from build123d import *

# Parameters (mm, degrees)
AUFSATZ_LINEAR_AUSTRAGEN1_DEPTH  = 67
SKIZZE3_W                        = 151
SKIZZE3_H                        = 2
AUFSATZ_LINEAR_AUSTRAGEN2_DEPTH  = 47.34238026
SKIZZE4_W                        = 2
SKIZZE4_H                        = 65
AUFSATZ_LINEAR_AUSTRAGEN3_DEPTH  = 47.39811
SKIZZE6_W                        = 149
SKIZZE6_H                        = 2
AUFSATZ_LINEAR_AUSTRAGEN4_DEPTH  = 47.40101983
SKIZZE7_W                        = 2
SKIZZE7_H                        = 63
AUFSATZ_LINEAR_AUSTRAGEN5_DEPTH  = 47.37320267
SKIZZE20_W                       = 147
SKIZZE20_H                       = 12.080237494
AUFSATZ_LINEAR_AUSTRAGEN6_DEPTH  = 63
SCHNITT_LINEAR_AUSTRAGEN1_DEPTH  = 137.764615455
SKIZZE23_W                       = 7.8
SKIZZE23_H                       = 5.4
SCHNITT_LINEAR_AUSTRAGEN12_DEPTH = 47
SKIZZE26_R                       = 2.05
SCHNITT_LINEAR_AUSTRAGEN13_DEPTH = 38
SKIZZE28_R                       = 2.05
SCHNITT_LINEAR_AUSTRAGEN14_DEPTH = 38
SCHNITT_LINEAR_START             = -38
SKIZZE29_R                       = 2.05
SCHNITT_LINEAR_AUSTRAGEN15_DEPTH = 38
SKIZZE31_R                       = 2.05
SCHNITT_LINEAR_AUSTRAGEN16_DEPTH = 38
SKIZZE32_R                       = 3
AUFSATZ_LINEAR_AUSTRAGEN15_DEPTH = 23.29
SKIZZE33_R                       = 3
AUFSATZ_LINEAR_AUSTRAGEN16_DEPTH = 23.29
SKIZZE34_R                       = 1.65
SCHNITT_LINEAR_AUSTRAGEN17_DEPTH = 25
SKIZZE35_R                       = 1.65
SCHNITT_LINEAR_AUSTRAGEN18_DEPTH = 25
SKIZZE37_W                       = 67
SKIZZE37_H                       = 9
SCHNITT_LINEAR_AUSTRAGEN20_DEPTH = 6.5
SKIZZE38_W                       = 67
SKIZZE38_H                       = 9
SCHNITT_LINEAR_AUSTRAGEN21_DEPTH = 6.5
FASE2_SIZE                       = 1
FASE13_SIZE                      = 1
SKIZZE40_R                       = 2.85
AUFSATZ_LINEAR_AUSTRAGEN17_DEPTH = 1.5
SKIZZE41_R                       = 1.65
SCHNITT_LINEAR_AUSTRAGEN23_DEPTH = 5
SKIZZE42_R                       = 2.85
AUFSATZ_LINEAR_AUSTRAGEN18_DEPTH = 1.5
SCHNITT_LINEAR_AUSTRAGEN24_DEPTH = 2
SKIZZE46_W                       = 5
SKIZZE46_H                       = 2.5
AUFSATZ_LINEAR_AUSTRAGEN21_DEPTH = 5
SKIZZE47_W                       = 5
SKIZZE47_H                       = 2.5
AUFSATZ_LINEAR_AUSTRAGEN22_DEPTH = 5
SKIZZE48_W                       = 38
SKIZZE48_H                       = 20.6
SCHNITT_LINEAR_AUSTRAGEN25_DEPTH = 2
SKIZZE49_W                       = 38
SKIZZE49_H                       = 2
AUFSATZ_LINEAR_AUSTRAGEN23_DEPTH = 10
SKIZZE51_R                       = 3
AUFSATZ_LINEAR_AUSTRAGEN24_DEPTH = 2.5
SKIZZE52_R                       = 1.6
SCHNITT_LINEAR_AUSTRAGEN26_DEPTH = 15


with BuildPart() as part:
    # Skizze1 → Aufsatz-Linear austragen1 (new body)
    with BuildSketch(Plane.XY):
        with BuildLine():
            Line((13.401569275, 0), (13.401569275, -2))
            Line((13.401569275, -2), (53.401569275, -2))
            Line((53.401569275, -2), (53.401569275, 0))
            ThreePointArc((53.401569275, 0), (63.401569275, 10), (73.401569275, 0))
            Line((73.401569275, 0), (73.401569275, -2))
            Line((73.401569275, -2), (109.401569275, -2))
            Line((109.401569275, -2), (109.401569275, 0))
            Line((109.401569275, 0), (75.401569275, 0))
            ThreePointArc((75.401569275, 0), (63.401569275, 12), (51.401569275, 0))
            Line((51.401569275, 0), (15.488199501, 0))
            ThreePointArc((15.488199501, 0), (3.901569275, 8.877501001), (-7.685060952, 0))
            Line((-7.685060952, 0), (-41.598430725, 0))
            Line((-41.598430725, 0), (-41.598430725, -2))
            Line((-41.598430725, -2), (-5.598430725, -2))
            Line((-5.598430725, -2), (-5.598430725, 0))
            ThreePointArc((-5.598430725, 0), (3.901569275, 6.877501001), (13.401569275, 0))
        make_face()
    extrude(amount=AUFSATZ_LINEAR_AUSTRAGEN1_DEPTH)

    # Skizze3 → Aufsatz-Linear austragen2 (add)
    with BuildSketch(Plane(origin=(0, 0, 0), x_dir=(1, 0, 0), z_dir=(0, 1, 0))):
        with Locations((33.901569275, -1)):
            Rectangle(SKIZZE3_W, SKIZZE3_H)
    extrude(amount=AUFSATZ_LINEAR_AUSTRAGEN2_DEPTH)

    # Skizze4 → Aufsatz-Linear austragen3 (add)
    with BuildSketch(Plane(origin=(0, 0, 0), x_dir=(1, 0, 0), z_dir=(0, 1, 0))):
        with Locations((-40.598430725, -34.5)):
            Rectangle(SKIZZE4_W, SKIZZE4_H)
    extrude(amount=AUFSATZ_LINEAR_AUSTRAGEN3_DEPTH)

    # Skizze6 → Aufsatz-Linear austragen4 (add)
    with BuildSketch(Plane(origin=(0, 0, 0), x_dir=(1, 0, 0), z_dir=(0, 1, 0))):
        with Locations((34.901569275, -66)):
            Rectangle(SKIZZE6_W, SKIZZE6_H)
    extrude(amount=AUFSATZ_LINEAR_AUSTRAGEN4_DEPTH)

    # Skizze7 → Aufsatz-Linear austragen5 (add)
    with BuildSketch(Plane(origin=(0, 0, 0), x_dir=(1, 0, 0), z_dir=(0, 1, 0))):
        with Locations((108.401569275, -33.5)):
            Rectangle(SKIZZE7_W, SKIZZE7_H)
    extrude(amount=AUFSATZ_LINEAR_AUSTRAGEN5_DEPTH)

    # Skizze20 → Aufsatz-Linear austragen6 (add)
    with BuildSketch(Plane.XY.offset(2)):
        with Locations((33.901569275, 6.040118747)):
            Rectangle(SKIZZE20_W, SKIZZE20_H)
    extrude(amount=AUFSATZ_LINEAR_AUSTRAGEN6_DEPTH)

    # Skizze8 → Schnitt-Linear austragen1 (cut, through all)
    with BuildSketch(Plane.XY.offset(67)):
        with BuildLine():
            Line((53.401569275, 0), (73.401569275, 0))
            ThreePointArc((73.401569275, 0), (63.401569275, 10), (53.401569275, 0))
        make_face()
        with BuildLine():
            Line((-5.598430725, 0), (13.401569275, 0))
            ThreePointArc((13.401569275, 0), (3.901569275, 9.5), (-5.598430725, 0))
        make_face()
    extrude(amount=-SCHNITT_LINEAR_AUSTRAGEN1_DEPTH, mode=Mode.SUBTRACT)

    # Skizze23 → Schnitt-Linear austragen12 (cut)
    with BuildSketch(Plane(origin=(109.401569275, 0, 0), x_dir=(0, 0, -1), z_dir=(1, 0, 0))):
        with Locations((-60.6, 17.280237494)):
            Rectangle(SKIZZE23_W, SKIZZE23_H)
        with Locations((-50.4, 17.280237494)):
            Rectangle(SKIZZE23_W, SKIZZE23_H)
    extrude(amount=-SCHNITT_LINEAR_AUSTRAGEN12_DEPTH, mode=Mode.SUBTRACT)

    # Skizze26 → Schnitt-Linear austragen13 (cut)
    with BuildSketch(Plane(origin=(109.401569275, 0, 0), x_dir=(0, 0, -1), z_dir=(1, 0, 0))):
        with Locations((-57, 3)):
            Circle(SKIZZE26_R)
    extrude(amount=-SCHNITT_LINEAR_AUSTRAGEN13_DEPTH, mode=Mode.SUBTRACT)

    # Skizze28 → Schnitt-Linear austragen14 (cut)
    with BuildSketch(Plane(origin=(109.401569275, 0, 0), x_dir=(0, 0, -1), z_dir=(1, 0, 0))):
        with Locations((-10, 3)):
            Circle(SKIZZE28_R)
    extrude(amount=-SCHNITT_LINEAR_AUSTRAGEN14_DEPTH, mode=Mode.SUBTRACT)

    # Skizze29 → Schnitt-Linear austragen15 (cut)
    with BuildSketch(Plane.ZY.offset(41.598430725).offset(SCHNITT_LINEAR_START)):
        with Locations(Location((57, 3, 0), (0, 0, 180))):
            Circle(SKIZZE29_R)
    extrude(amount=SCHNITT_LINEAR_AUSTRAGEN15_DEPTH, mode=Mode.SUBTRACT)

    # Skizze31 → Schnitt-Linear austragen16 (cut)
    with BuildSketch(Plane.ZY.offset(41.598430725).offset(SCHNITT_LINEAR_START)):
        with Locations(Location((10, 3, 0), (0, 0, 180))):
            Circle(SKIZZE31_R)
    extrude(amount=SCHNITT_LINEAR_AUSTRAGEN16_DEPTH, mode=Mode.SUBTRACT)

    # Skizze32 → Aufsatz-Linear austragen15 (add)
    with BuildSketch(Plane(origin=(0, 12.080237494, 0), x_dir=(1, 0, 0), z_dir=(0, 1, 0))):
        with Locations((-36.098430725, -61.5)):
            Circle(SKIZZE32_R)
    extrude(amount=AUFSATZ_LINEAR_AUSTRAGEN15_DEPTH)

    # Skizze33 → Aufsatz-Linear austragen16 (add)
    with BuildSketch(Plane(origin=(0, 12.080237494, 0), x_dir=(1, 0, 0), z_dir=(0, 1, 0))):
        with Locations((103.901569275, -5.5)):
            Circle(SKIZZE33_R)
    extrude(amount=AUFSATZ_LINEAR_AUSTRAGEN16_DEPTH)

    # Skizze34 → Schnitt-Linear austragen17 (cut)
    with BuildSketch(Plane(origin=(0, 35.370237494, 0), x_dir=(1, 0, 0), z_dir=(0, 1, 0))):
        with Locations(Location((-36.098430725, -61.5, 0), (0, 0, 180))):
            Circle(SKIZZE34_R)
    extrude(amount=-SCHNITT_LINEAR_AUSTRAGEN17_DEPTH, mode=Mode.SUBTRACT)

    # Skizze35 → Schnitt-Linear austragen18 (cut)
    with BuildSketch(Plane(origin=(0, 35.370237494, 0), x_dir=(1, 0, 0), z_dir=(0, 1, 0))):
        with Locations(Location((103.901569275, -5.5, 0), (0, 0, 180))):
            Circle(SKIZZE35_R)
    extrude(amount=-SCHNITT_LINEAR_AUSTRAGEN18_DEPTH, mode=Mode.SUBTRACT)

    # Skizze37 → Schnitt-Linear austragen20 (cut)
    with BuildSketch(Plane(origin=(109.401569275, 0, 0), x_dir=(0, 0, -1), z_dir=(1, 0, 0))):
        with Locations((-33.5, 2.5)):
            Rectangle(SKIZZE37_W, SKIZZE37_H)
    extrude(amount=-SCHNITT_LINEAR_AUSTRAGEN20_DEPTH, mode=Mode.SUBTRACT)

    # Skizze38 → Schnitt-Linear austragen21 (cut)
    with BuildSketch(Plane.ZY.offset(41.598430725)):
        with Locations((33.5, 2.5)):
            Rectangle(SKIZZE38_W, SKIZZE38_H)
    extrude(amount=-SCHNITT_LINEAR_AUSTRAGEN21_DEPTH, mode=Mode.SUBTRACT)

    # Fase2
    fase2_edges = [part.edges().sort_by_distance(p)[0] for p in [
        (-41.598430725, 27.17119013, 0),
        (109.401569275, 27.17119013, 0),
        (109.401569275, 27.200509915, 67),
        (109.401569275, 7, 33.5),
        (102.901569275, 2.5, 67),
        (106.151569275, 7, 67),
        (102.901569275, 2.5, 0),
        (106.151569275, 7, 0),
        (102.901569275, -2, 33.5),
        (-41.598430725, 7, 33.5),
        (-35.098430725, 2.5, 0),
        (-38.348430725, 7, 0),
        (-35.098430725, 2.5, 67),
        (-38.348430725, 7, 67),
        (-35.098430725, -2, 33.5),
        (-41.598430725, 27.199055, 67),
    ]]
    chamfer(fase2_edges, length=FASE2_SIZE)

    # Fase13
    fase13_edges = [part.edges().sort_by_distance(p)[0] for p in [
        (33.401569275, -2, 67),
        (87.651569275, -2, 0),
        (33.401569275, -2, 0),
        (87.651569275, -2, 67),
        (-19.848430725, -2, 0),
        (-19.848430725, -2, 67),
    ]]
    chamfer(fase13_edges, length=FASE13_SIZE)

    # Skizze40 → Aufsatz-Linear austragen17 (add)
    with BuildSketch(Plane(origin=(0, 12.080237494, 0), x_dir=(1, 0, 0), z_dir=(0, 1, 0))):
        with Locations((103.091569275, -37.57)):
            Circle(SKIZZE40_R)
    extrude(amount=AUFSATZ_LINEAR_AUSTRAGEN17_DEPTH)

    # Skizze41 → Schnitt-Linear austragen23 (cut)
    with BuildSketch(Plane(origin=(0, 13.580237494, 0), x_dir=(1, 0, 0), z_dir=(0, 1, 0))):
        with Locations(Location((103.091569275, -37.59, 0), (0, 0, 180))):
            Circle(SKIZZE41_R)
    extrude(amount=-SCHNITT_LINEAR_AUSTRAGEN23_DEPTH, mode=Mode.SUBTRACT)

    # Skizze42 → Aufsatz-Linear austragen18 (add)
    with BuildSketch(Plane(origin=(0, 12.080237494, 0), x_dir=(1, 0, 0), z_dir=(0, 1, 0))):
        with Locations((103.091569275, -60.69)):
            Circle(SKIZZE42_R)
        with Locations((68.201569275, -60.69)):
            Circle(SKIZZE42_R)
    extrude(amount=AUFSATZ_LINEAR_AUSTRAGEN18_DEPTH)

    # Skizze43 → Schnitt-Linear austragen24 (cut)
    with BuildSketch(Plane(origin=(109.401569275, 0, 0), x_dir=(0, 0, -1), z_dir=(1, 0, 0))):
        with BuildLine():
            Line((-12.5, 19.780237494), (-10.5, 19.780237494))
            ThreePointArc((-10.5, 19.780237494), (-8, 17.280237494), (-10.5, 14.780237494))
            Line((-10.5, 14.780237494), (-12.5, 14.780237494))
            ThreePointArc((-12.5, 14.780237494), (-15, 17.280237494), (-12.5, 19.780237494))
        make_face()
    extrude(amount=-SCHNITT_LINEAR_AUSTRAGEN24_DEPTH, mode=Mode.SUBTRACT)

    # Skizze46 → Aufsatz-Linear austragen21 (add)
    with BuildSketch(Plane(origin=(-39.598430725, 0, 0), x_dir=(0, 0, -1), z_dir=(1, 0, 0))):
        with Locations((-4.5, 34.120237494)):
            Rectangle(SKIZZE46_W, SKIZZE46_H)
    extrude(amount=AUFSATZ_LINEAR_AUSTRAGEN21_DEPTH)

    # Skizze47 → Aufsatz-Linear austragen22 (add)
    with BuildSketch(Plane.ZY.offset(-107.401569275)):
        with Locations((62.5, 34.120237494)):
            Rectangle(SKIZZE47_W, SKIZZE47_H)
    extrude(amount=AUFSATZ_LINEAR_AUSTRAGEN22_DEPTH)

    # Skizze48 → Schnitt-Linear austragen25 (cut)
    with BuildSketch(Plane.ZY.offset(41.598430725)):
        with Locations((33.5, 24.82)):
            Rectangle(SKIZZE48_W, SKIZZE48_H)
    extrude(amount=-SCHNITT_LINEAR_AUSTRAGEN25_DEPTH, mode=Mode.SUBTRACT)

    # Skizze49 → Aufsatz-Linear austragen23 (add)
    with BuildSketch(Plane.ZY.offset(41.598430725)):
        with Locations((33.5, 13.52)):
            Rectangle(SKIZZE49_W, SKIZZE49_H)
    extrude(amount=AUFSATZ_LINEAR_AUSTRAGEN23_DEPTH)

    # Skizze51 → Aufsatz-Linear austragen24 (add)
    with BuildSketch(Plane(origin=(0, 12.080237494, 0), x_dir=(1, 0, 0), z_dir=(0, 1, 0))):
        with Locations((-9.198430725, -29)):
            Circle(SKIZZE51_R)
    extrude(amount=AUFSATZ_LINEAR_AUSTRAGEN24_DEPTH)

    # Skizze52 → Schnitt-Linear austragen26 (cut)
    with BuildSketch(Plane(origin=(0, 14.580237494, 0), x_dir=(1, 0, 0), z_dir=(0, 1, 0))):
        with Locations(Location((-9.198430725, -29, 0), (0, 0, 180))):
            Circle(SKIZZE52_R)
    extrude(amount=-SCHNITT_LINEAR_AUSTRAGEN26_DEPTH, mode=Mode.SUBTRACT)


solid = part.part
Work out the finished part from the listing and answer in its coordinate system (mm). A direction names the side the tool comes from. Give positions to 0.01 mm unless a question says otherwise; leave off trailing zeros. Order: outer loops, then holes, each group sorted by start corner. A loop starts at its lowest first (then second) coordinate and runs counter-clockwise, first axis right, second up. Notation, with made-up numbers: (33.25, 76) -> (45.25, 76) arc R11 cw to (45.25, 88) -> close; hole circle Ø8 at (5, 35.25). An arc over 180 degrees is marked (long way). Answer as a JSON object with one key per item and string values. Group by question number.
1. Section B-B on z = 51 is taken. Count the separate pieces of the cut face and the enclosed holes in it, plus the area to 3 significant figures.
2. The mould has two halves that part along Y. Classify faces 6 (the flat face through (-46, 14.52, 33)), 7 (the flat face through (-36, 10.37, 62)), 8 (the cylindrical face through (100.904, 23.562, 5.368)): released by +Y, released by -Y, zero draft, split by the parting line, or undercut.
3. A tool of negligible diameter and unlimited length cuts with its end or side. For faces 1 (the flat face through (-37, 32.87, 5)), 2 (the flat face through (-20, -2, 33)), 3 (the cylindrical face through (63.6, 10, 34)), 4 (the flat face through (106, 7, 34)), 5 (the flat face through (103, 8.58, 38)), from which of +Z, -Z, +X, -X, +Y, -Y can it reach the whole face along a straight path? Write none if from no direction.
4. Flat-ended cylindrical pins translate along their axes: pin 1 Ø5 at (x, z) = (-36.5, 61.5) entering from +Y; pin 2 Ø2 at (x, z) = (108, 62) entering from -Y; pin 3 Ø2.5 at (y, z) = (3, 10) entering from +X. Find the tip coordinate at first contact, or state that the pin passes through.
5. Consider line 1 along Z through (x, y) = (92, 3); line 2 along Z through (x, y) = (45, 40.5); line 3 along X through (y, z) = (13.5, 59.5). Determine where each line is inside the solid, lowest interval first. Write a range as [from, to].
6. Section A-A on y = 25 is taken. Determine the outline of the cut face in (x, z), plus the area to 3 significant figures.
7. Section D-D on x = 37 is taken. Determine the outline of the cut face in (y, z), plus the area to 3 significant figures.
Result sheet:
{
 "1": {"separate pieces": "3", "enclosed holes": "0", "area": "1,740 mm^2"},
 "2": {"face 6": "undercut", "face 7": "released by +Y", "face 8": "zero draft"},
 "3": {"face 1": "none", "face 2": "+Z, -Z, +X, -X, -Y", "face 3": "+Z, -Z, -Y", "face 4": "+Z, -Z, +X, -Y", "face 5": "+Y"},
 "4": {"pin 1": "stops at y = 35.37", "pin 2": "stops at y = 7", "pin 3": "stops at x = 54.35"},
 "5": {"line 1": "z = [0, 7.95], [12.05, 54.95], [59.05, 67]", "line 2": "z = [0, 2], [65, 67]", "line 3": "x = [-41.6, -39.6], [-38.33, -33.86], [65.61, 70.79], [100.5, 105.68], [107.4, 109.4]"},
 "6": {"outline": "(-41.6, 1) -> (-40.6, 0) -> (108.4, 0) -> (109.4, 1) -> (109.4, 66) -> (108.4, 67) -> (-40.6, 67) -> (-41.6, 66) -> (-41.6, 52.5) -> (-39.6, 52.5) -> (-39.6, 65) -> (107.4, 65) -> (107.4, 2) -> (-39.6, 2) -> (-39.6, 14.5) -> (-41.6, 14.5) -> close; circle Ø6 at (-36.1, 61.5); circle Ø6 at (103.9, 5.5); hole circle Ø3.3 at (-36.1, 61.5); hole circle Ø3.3 at (103.9, 5.5)", "area": "817 mm^2"},
 "7": {"outline": "(-2, 1) -> (-1, 0) -> (47.34, 0) -> (47.34, 2) -> (12.08, 2) -> (12.08, 65) -> (47.4, 65) -> (47.4, 67) -> (-1, 67) -> (-2, 66) -> close", "area": "1,080 mm^2"}
}
